Can you work these out from the model? Positions are in its coordinate system, mm. A direction names the side the tool comes from. Give positions to 0.01 mm unless a question says otherwise; leave off trailing zeros. Write each loop counter-clockwise with the first axis right and the second up, starting at its lowest first coordinate (ties: lowest second). Pieces come first, ordered by that corner, then holes. Notation, with made-up numbers: (25.25, 54.25) -> (56.25, 54.25) arc R11 cw to (56.25, 60.25) -> close; hole circle Ø3 at (69, -24). An arc over 180 degrees is marked (long way). Answer as CSV lines item,"result". Start each with the question number.
1. I'm going to push flat-ended pins straight in: P1, Ø1.8, axis at x = -21, y = -2.5, coming from the +Z side; P2, Ø12, axis at x = -11.5, z = 12, coming from the +Y side; P3, Ø4, axis at x = 4, z = 9.5, coming from the -Y side; P4, Ø2, axis at x = 2, y = 4, coming from the +Z side. Where does each tip first touch, or does it pass through?
2. If we section it at A-A on y = 12.75: Write out the boundary of the cut face in (x, z).
3. If we section it at D-D on x = -13.3: Count the separate pieces of the cut face and the enclosed holes in it, plus the area to 3 significant figures.
4. On a 3-axis mill with a long thin cutter (end or side, diameter ignored), from which of +Z, -Z, +X, -X, +Y, -Y can I reach the whole of each face in a straight line? I mean faces 4 (the face through (-26, 6.5, -5)), 5 (the face through (-6, 1.5, 5)), 6 (the face through (-6, -17, -3)). Say none if no direction works.
5. If we section it at B-B on x = -20.5: Write out the boundary of the cut face in (y, z), plus the area to 3 significant figures.
6. If we section it at C-C on z = 10.5: Write out the boundary of the cut face in (x, y).
7. If we mould it in two halves opening along Y, with no side actions, what happens to faces 1 (the face through (-18, 24.5, -5)), 2 (the face through (-6, -24.5, -1)), 3 (the face through (8.272, -12.265, -1.479))? For each: pulls with the +Y half, pulls with the -Y half, needs draft (parallel to the pull), parting line crosses it, or undercut.
8. I need wall thicknesses on line 1 (Y direction, x = -20.5, z = -1.4); line 2 (Y direction, x = -13.3, z = -4.05); line 3 (Y direction, x = -13.3, z = -4.15). Which ranges of each line are inside material? Lowest first, please. Write a range as [from, to].
```python
from build123d import *

# Parameters (mm, degrees)
SKETCH_5_R              = 1.75
EXTRUDE_15981_DEPTH     = 3
EXTRUDE_2_DEPTH         = 15
EXTRUDE_2_DEPTH_BACK    = 5.8
SKETCH_6_W              = 49
SKETCH_6_H              = 8
EXTRUDE_START           = -5.8
SKETCH_7_R              = 1.5
SKETCH_7_R_2            = 7.75
EXTRUDE_3_DEPTH         = 2
CUT_EXTRUDE_START       = 15
SKETCH_9_R              = 1.15
CUT_EXTRUDE_16680_DEPTH = 10
CHAMFER_16885_SIZE      = 3
CHAMFER_16885_SIZE_2    = 3.8
FILLET_16929_R          = 3


with BuildPart() as part:
    # Sketch 5 → Extrude 15981 (new body)
    with BuildSketch(Plane.XY):
        Polygon((18.5, -24.5), (18.5, -6.5), (-30.5, -6.5), (-30.5, -24.5), (-18.5, -24.5), align=None)
        with Locations((-20.5, -14)):
            Circle(SKETCH_5_R, mode=Mode.SUBTRACT)
        with Locations((8.5, -14)):
            Circle(SKETCH_5_R, mode=Mode.SUBTRACT)
    extrude(amount=-EXTRUDE_15981_DEPTH)

    # Эскиз внешнего крепления двигателя колеса<6> → Extrude 2 (add, two sides: drawn at the far end of the back side and taken through both)
    with BuildSketch(Plane.XY.offset(-EXTRUDE_2_DEPTH_BACK)):
        with Locations((-6, -2.5)):
            Rectangle(SKETCH_6_W, SKETCH_6_H)
    extrude(amount=EXTRUDE_2_DEPTH + EXTRUDE_2_DEPTH_BACK)

    # Sketch 7 → Extrude 3 (add)
    with BuildSketch(Plane.XY.offset(EXTRUDE_START)):
        with BuildLine():
            ThreePointArc((-9.945898034, 24.5), (-13.3, 26), (-16.654101966, 24.5))
            Line((-16.654101966, 24.5), (-18.5, 24.5))
            Line((-18.5, 24.5), (-18.5, 20))
            Line((-18.5, 20), (-21.5, 20))
            Line((-21.5, 20), (-21.5, 6.5))
            Line((-21.5, 6.5), (-30.5, 6.5))
            Line((-30.5, 6.5), (-30.5, 1.5))
            Line((-30.5, 1.5), (18.5, 1.5))
            Line((18.5, 1.5), (18.5, 24.5))
            Line((18.5, 24.5), (-9.945898034, 24.5))
        make_face()
        with Locations((-13.3, 4)):
            Circle(SKETCH_7_R, mode=Mode.SUBTRACT)
        with Locations((-13.3, 21.5)):
            Circle(SKETCH_7_R, mode=Mode.SUBTRACT)
        with Locations((7.3, 12.75)):
            Circle(SKETCH_7_R_2, mode=Mode.SUBTRACT)
    extrude(amount=EXTRUDE_3_DEPTH)

    # Sketch 9 → Cut-Extrude 16680 (cut)
    with BuildSketch(Plane.XY.offset(CUT_EXTRUDE_START)):
        with Locations((8.5, -2.5)):
            Circle(SKETCH_9_R)
        with Locations((-20.5, -2.5)):
            Circle(SKETCH_9_R)
    extrude(amount=-CUT_EXTRUDE_16680_DEPTH, mode=Mode.SUBTRACT)

    # Chamfer 16786: read off the stored shape, not the designer's step
    # Chamfer 16786: loft between two sections, ruled curve by curve
    chamfer_16786_from = [
        Edge.make_three_point_arc((-11.8, 4, -4.3), (-13.3, 2.5, -4.3), (-14.8, 4, -4.3)),
        Edge.make_three_point_arc((-14.8, 4, -4.3), (-13.3, 5.5, -4.3), (-11.8, 4, -4.3)),
    ]
    chamfer_16786_to = [
        Edge.make_three_point_arc((-10.7, 4, -5.8), (-13.3, 1.4, -5.8), (-15.9, 4, -5.8)),
        Edge.make_three_point_arc((-15.9, 4, -5.8), (-13.3, 6.6, -5.8), (-10.7, 4, -5.8)),
    ]
    chamfer_16786 = Solid(Shell([*[Face.make_surface_from_curves(chamfer_16786_from[k], chamfer_16786_to[k]) for k in range(2)], Face(Wire(chamfer_16786_from)), Face(Wire(chamfer_16786_to))]))
    add(chamfer_16786, mode=Mode.SUBTRACT)

    # Chamfer 16786 2: loft between two sections, ruled curve by curve
    chamfer_16786_2_from = [
        Edge.make_three_point_arc((-11.8, 21.5, -4.3), (-13.3, 20, -4.3), (-14.8, 21.5, -4.3)),
        Edge.make_three_point_arc((-14.8, 21.5, -4.3), (-13.3, 23, -4.3), (-11.8, 21.5, -4.3)),
    ]
    chamfer_16786_2_to = [
        Edge.make_three_point_arc((-10.7, 21.5, -5.8), (-13.3, 18.9, -5.8), (-15.9, 21.5, -5.8)),
        Edge.make_three_point_arc((-15.9, 21.5, -5.8), (-13.3, 24.1, -5.8), (-10.7, 21.5, -5.8)),
    ]
    chamfer_16786_2 = Solid(Shell([*[Face.make_surface_from_curves(chamfer_16786_2_from[k], chamfer_16786_2_to[k]) for k in range(2)], Face(Wire(chamfer_16786_2_from)), Face(Wire(chamfer_16786_2_to))]))
    add(chamfer_16786_2, mode=Mode.SUBTRACT)

    # Chamfer 16885
    # the kernel refuses this chamfer: 3.8, 3 mm, written as the material it adds along each edge
    with BuildSketch(Plane(origin=(18.5, -6.5, -3), x_dir=(0, -1, 0), z_dir=(-1, 0, 0))) as chamfer_16885_piece_1_section:
        Polygon((CHAMFER_16885_SIZE, 0), (0, -CHAMFER_16885_SIZE_2), (0, 0), align=None)
    chamfer_16885_piece_1 = extrude(amount=49, mode=Mode.PRIVATE)
    chamfer_16885_piece_1 = split(chamfer_16885_piece_1, bisect_by=Plane(origin=(18.5, -6.5, -5.8), z_dir=(0, 0, 1)), keep=Keep.TOP, mode=Mode.PRIVATE)
    add(chamfer_16885_piece_1)

    # Fillet 16929
    fillet_16929_edges = [part.edges().sort_by_distance(p)[0] for p in [
        (18.5, 24.5, -4.8),
    ]]
    fillet(fillet_16929_edges, radius=FILLET_16929_R)


solid = part.part
```
Computed values:
1,P1,"stops at z = 15"
1,P2,"stops at y = 1.5"
1,P3,"stops at y = -6.5"
1,P4,"stops at z = -3.8"
2,outline,"(-21.5, -5.8) -> (-0.45, -5.8) -> (-0.45, -3.8) -> (-21.5, -3.8) -> close; (15.05, -5.8) -> (18.5, -5.8) -> (18.5, -3.8) -> (15.05, -3.8) -> close"
3,separate pieces,"3"
3,enclosed holes,"0"
3,area,"259 mm2"
4,face 4,"+Z, -Z, -X, +Y"
4,face 5,"+Z, +X, -X, +Y"
4,face 6,"-Z, +X, -X, -Y"
5,outline,"(-24.5, -3) -> (-15.75, -3) -> (-15.75, 0) -> (-24.5, 0) -> close; (-12.25, -3) -> (-9.5, -3) -> (-7.29, -5.8) -> (20, -5.8) -> (20, -3.8) -> (1.5, -3.8) -> (1.5, 15) -> (-1.35, 15) -> (-1.35, 5) -> (-3.65, 5) -> (-3.65, 15) -> (-6.5, 15) -> (-6.5, 0) -> (-12.25, 0) -> close"
5,area,"229 mm2"
6,outline,"(-30.5, -6.5) -> (18.5, -6.5) -> (18.5, 1.5) -> (-30.5, 1.5) -> close; hole circle Ø2.3 at (-20.5, -2.5); hole circle Ø2.3 at (8.5, -2.5)"
7,face 1,"pulls with the +Y half"
7,face 2,"pulls with the -Y half"
7,face 3,"undercut"
8,line 1,"y = [-24.5, -15.75], [-12.25, 1.5]"
8,line 2,"y = [-8.67, 2.5], [5.5, 20], [23, 26]"
8,line 3,"y = [-8.59, 2.5], [5.5, 20], [23, 26]"
